```python
from build123d import *

# Parameters (mm, degrees)
ESBO_O1_R                       = 39.125
RESSALTO_EXTRUS_O1_DEPTH        = 128
FURO_ROSCADO_DE_M51_D           = 4.2
FURO_ROSCADO_DE_M51_DEPTH       = 10
FURO_ROSCADO_DE_M51_CSINK_D     = 5.05
FURO_ROSCADO_DE_M51_CSINK_ANGLE = 90
FURO_ROSCADO_DE_M51_TIP         = 1.2618073
ESBO_O1_4_R                     = 6
RESSALTO_EXTRUS_O2_DEPTH        = 25


with BuildPart() as part:
    # Esboço1 → Ressalto-extrusão1 (new body)
    with BuildSketch(Plane.XY):
        Circle(ESBO_O1_R)
    extrude(amount=RESSALTO_EXTRUS_O1_DEPTH)

    # Furo roscado de M51
    with Locations(Plane(origin=(0, 0, 0), x_dir=(-1, 0, 0), z_dir=(0, 0, -1))):
        with Locations((0, 26), (-26, 0), (0, -26), (26, 0)):
            CounterSinkHole(FURO_ROSCADO_DE_M51_D / 2, FURO_ROSCADO_DE_M51_CSINK_D / 2, depth=FURO_ROSCADO_DE_M51_DEPTH, counter_sink_angle=FURO_ROSCADO_DE_M51_CSINK_ANGLE)
            with Locations((0, 0, -(FURO_ROSCADO_DE_M51_DEPTH + FURO_ROSCADO_DE_M51_TIP / 2))):  # 118° drill point
                Cone(0, FURO_ROSCADO_DE_M51_D / 2, FURO_ROSCADO_DE_M51_TIP, mode=Mode.SUBTRACT)

    # Esboço1<4> → Ressalto-extrusão2 (add)
    with BuildSketch(Plane.XY):
        Circle(ESBO_O1_4_R)
    extrude(amount=-RESSALTO_EXTRUS_O2_DEPTH)


solid = part.part
```
Source: CAD feature listing. Evaluate the final solid. Frame: model axes, mm. A direction names the side the tool comes from. Give positions to 0.01 mm unless a question says otherwise; leave off trailing zeros. Order: outer loops, then holes, each group sorted by start corner. A loop starts at its lowest first (then second) coordinate and runs counter-clockwise, first axis right, second up.
(1) Material intervals for line 1 along Y through (x, z) = (0, 6) (3 decimals); line 2 along Z through (x, y) = (28.5, 19.5); line 3 along X through (y, z) = (-26, 4.25), sorted ascending.
(2) Section query B-B (x = 11). Return the cut outline in (y, z), plus the area to 3 significant figures.
(3) Section query A-A (z = 29). Return the cut outline in (x, y) (3 decimals), plus the area to 3 significant figures.
(4) Section query C-C (y = -14). Return the cut outline in (x, z), plus the area to 3 significant figures.
(5) Access query for faces 1 (the face through (23.9, 0.09, 5.28)), 2 (the face through (21.033, 32.99, 63.104)). Directions: +Z, -Z, +X, -X, +Y, -Y. A direction counts if a zero-diameter tool reaches every point of the face in a straight line with its end or side. Return the directions, or none.
(6) Contact query for flat-ended pins moving along their axis: P1, Ø1.5, axis at y = 17.5, z = 86.5, coming from the +X side; P2, Ø10, axis at y = 29.5, z = 98.5, coming from the -X side; P3, Ø4, axis at x = -26, y = 0, coming from the -Z side. Output: stop coordinate, or through.
(7) Pull-direction query (Y, two-part tool) for faces 3 (the face through (-6, 0, -12)), 4 (the face through (-1, 1, 128)), 5 (the face through (1.13, -24.23, 5.28)); classes: +Y half, -Y half, draft (parallel to the pull), parting line (faces both ways), or undercut.
Outcome:
1. line 1: y = -39.125 to -28.1, -23.9 to 23.9, 28.1 to 39.125
1. line 2: z = 0 to 128
1. line 3: x = -29.24 to -2.1, 2.1 to 29.24
2. outline: (-37.55, 0) - (37.55, 0) - (37.55, 128) - (-37.55, 128) - close
2. area: 9,610 mm2
3. outline: circle Ø78.25 at (0, 0)
3. area: 4,810 mm2
4. outline: (-36.53, 0) - (36.53, 0) - (36.53, 128) - (-36.53, 128) - close
4. area: 9,350 mm2
5. face 1: -Z
5. face 2: +Z, -Z
6. P1: stops at x = 35.36
6. P2: stops at x = -30.5
6. P3: stops at z = 10.06
7. face 3: parting line
7. face 4: draft
7. face 5: undercut
